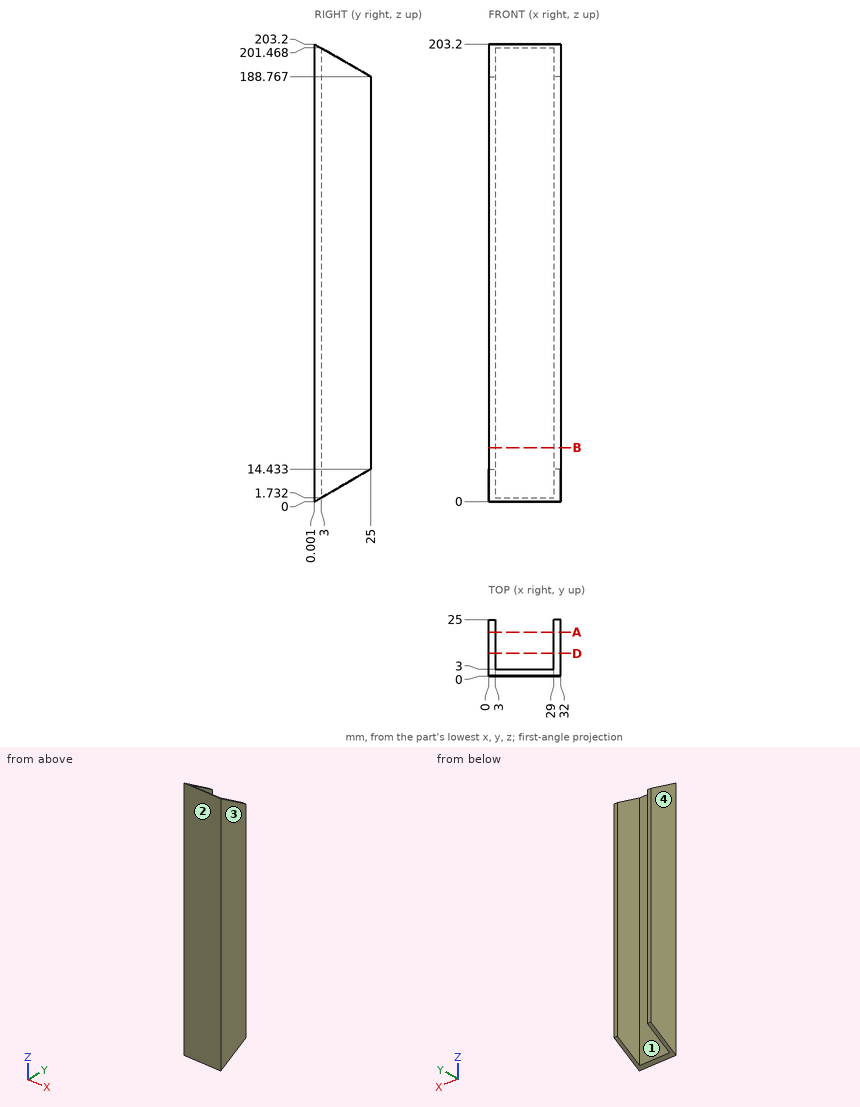
Answer from the drawing. Dimensions are ordinates in mm from the lowest x, y and z of the part. Give positions to 0.01 mm unless a question says otherwise; leave off trailing zeros. Order: outer loops, then holes, each group sorted by start corner. A loop starts at its lowest first (then second) coordinate and runs counter-clockwise, first axis right, second up. Notation, with made-up numbers: (-9.75, -39.75) -> (29.25, -39.75) arc R28 cw to (29.25, -20.75) -> close; hole circle Ø7 at (-16, -4.75). An arc over 180 degrees is marked (long way). One line per item, written item: value. Start each with the question number.
(1) For a pull along X with two mould halves and no side action, classify the marked faces 1, 2, 3 and 4 as released by +X, released by -X, zero draft, split by the parting line, or undercut.
(2) The part is cut by section A-A (y = 19.5). Determine the outline of the cut face in (x, z), and give its area (3 significant figures).
(3) The part is cut by section B-B (z = 24). Determine the outline of the cut face in (x, y), and give its area (3 significant figures).
(4) Straight lines are drawn through the part: L1, parallel to X at y = 8, z = 24.5; L2, parallel to Y at x = 7, z = 115.5; L3, parallel to Z at x = 2, y = 24 (1 decimal). For each, find the intervals that lie inside material, in ascending order.
(5) The part is cut by section D-D (y = 10). Determine the outline of the cut face in (x, z), and give its area (3 significant figures).
(6) Flat-ended cylindrical pins translate along their axes: P1, Ø1.5, axis at x = 7.5, z = 75.5, coming from the +Y side; P2, Ø6, axis at x = 22, y = 8, coming from the +Z side. Find the tip coordinate at first contact, or state that the pin passes through.
Taken from the geometry:
1. face 1: undercut
1. face 2: zero draft
1. face 3: released by +X
1. face 4: released by -X
2. outline: (0, 11.26) -> (3, 11.26) -> (3, 191.94) -> (0, 191.94) -> close; (29, 11.26) -> (32, 11.26) -> (32, 191.94) -> (29, 191.94) -> close
2. area: 1,080 mm^2
3. outline: (0, 0) -> (32, 0) -> (32, 25) -> (29, 25) -> (29, 3) -> (3, 3) -> (3, 25) -> (0, 25) -> close
3. area: 228 mm^2
4. L1: 0 to 3, 29 to 32
4. L2: 0 to 3
4. L3: 13.9 to 189.3
5. outline: (0, 5.77) -> (3, 5.77) -> (3, 197.43) -> (0, 197.43) -> close; (29, 5.77) -> (32, 5.77) -> (32, 197.43) -> (29, 197.43) -> close
5. area: 1,150 mm^2
6. P1: y = 3
6. P2: through
